```python
from build123d import *

# Parameters (mm, degrees)
BOSS_EXTRUDE1_DEPTH = 65
BOSS_EXTRUDE3_START = -60
SKETCH2_R           = 50
SKETCH2_R_2         = 48
BOSS_EXTRUDE3_DEPTH = 100
CUT_EXTRUDE1_START  = -50
SKETCH2_6_R         = 48
CUT_EXTRUDE1_DEPTH  = 50
BOSS_EXTRUDE6_START = 50
SKETCH2_9_W         = 57.5
SKETCH2_9_H         = 81
SKETCH2_9_W_2       = 53.5
SKETCH2_9_H_2       = 77
BOSS_EXTRUDE6_DEPTH = 100
SKETCH2_10_W        = 53.5
SKETCH2_10_H        = 77
CUT_EXTRUDE2_DEPTH  = 50
SKETCH2_11_W        = 82
SKETCH2_11_H        = 81
SKETCH2_11_W_2      = 78
SKETCH2_11_H_2      = 77
SKETCH2_11_W_3      = 57.5
SKETCH2_11_W_4      = 53.5
SKETCH2_11_R        = 50
SKETCH2_11_R_2      = 48
BOSS_EXTRUDE7_DEPTH = 35
CUT_EXTRUDE4_DEPTH  = 3
SKETCH10_W          = 139.5
SKETCH10_H          = 50
BOSS_EXTRUDE9_DEPTH = 65
SKETCH10_3_W        = 139.5
SKETCH10_3_H        = 50
CUT_EXTRUDE5_DEPTH  = 20
SKETCH7_W           = 139.5
SKETCH7_H           = 50
BOSS_EXTRUDE8_DEPTH = 65
SKETCH8_W           = 135.5
SKETCH8_H           = 65
CUT_EXTRUDE6_DEPTH  = 30


with BuildPart() as part:
    # Sketch1 → Boss-Extrude1 (new body)
    with BuildSketch(Plane(origin=(0, 0, 0), x_dir=(1, 0, 0), z_dir=(0, 1, 0))):
        with BuildLine():
            Line((-70, -50), (120, -50))
            Line((120, -50), (120, 50))
            Line((120, 50), (-71, 50))
            ThreePointArc((-71, 50), (-105.648232278, 35.648232278), (-120, 1))
            Line((-120, 1), (-120, 0))
            ThreePointArc((-120, 0), (-105.355339059, -35.355339059), (-70, -50))
        make_face()
    extrude(amount=BOSS_EXTRUDE1_DEPTH)

    # Sketch2 → Boss-Extrude3 (add)
    with BuildSketch(Plane(origin=(0, 65, 0), x_dir=(1, 0, 0), z_dir=(0, 1, 0)).offset(BOSS_EXTRUDE3_START)):
        with Locations(Location((-70, 0, 0), (0, 0, 270))):
            Circle(SKETCH2_R)
        with Locations(Location((-70, 0, 0), (0, 0, 270))):
            Circle(SKETCH2_R_2, mode=Mode.SUBTRACT)
    extrude(amount=BOSS_EXTRUDE3_DEPTH)

    # Sketch2_6 → Cut-Extrude1 (cut)
    with BuildSketch(Plane(origin=(0, 65, 0), x_dir=(1, 0, 0), z_dir=(0, 1, 0)).offset(CUT_EXTRUDE1_START)):
        with Locations(Location((-70, 0, 0), (0, 0, 270))):
            Circle(SKETCH2_6_R)
    extrude(amount=CUT_EXTRUDE1_DEPTH, mode=Mode.SUBTRACT)

    # Sketch2_9 → Boss-Extrude6 (add)
    with BuildSketch(Plane(origin=(0, 65, 0), x_dir=(1, 0, 0), z_dir=(0, 1, 0)).offset(BOSS_EXTRUDE6_START)):
        with Locations((9.25, 9.5)):
            Rectangle(SKETCH2_9_W, SKETCH2_9_H)
        with Locations((9.25, 9.5)):
            Rectangle(SKETCH2_9_W_2, SKETCH2_9_H_2, mode=Mode.SUBTRACT)
    extrude(amount=-BOSS_EXTRUDE6_DEPTH)

    # Sketch2_10 → Cut-Extrude2 (cut)
    with BuildSketch(Plane(origin=(0, 65, 0), x_dir=(1, 0, 0), z_dir=(0, 1, 0))):
        with Locations((9.25, 9.5)):
            Rectangle(SKETCH2_10_W, SKETCH2_10_H)
    extrude(amount=-CUT_EXTRUDE2_DEPTH, mode=Mode.SUBTRACT)

    # Sketch2_11 → Boss-Extrude7 (add)
    # profile 1 of 3: a face of its own
    with BuildSketch(Plane(origin=(0, 65, 0), x_dir=(1, 0, 0), z_dir=(0, 1, 0))):
        with Locations((79, 9.5)):
            Rectangle(SKETCH2_11_W, SKETCH2_11_H)
        with Locations((79, 9.5)):
            Rectangle(SKETCH2_11_W_2, SKETCH2_11_H_2, mode=Mode.SUBTRACT)
    # profile 2 of 3: a face of its own
    with BuildSketch(Plane(origin=(0, 65, 0), x_dir=(1, 0, 0), z_dir=(0, 1, 0))):
        with Locations((9.25, 9.5)):
            Rectangle(SKETCH2_11_W_3, SKETCH2_11_H)
        with Locations((9.25, 9.5)):
            Rectangle(SKETCH2_11_W_4, SKETCH2_11_H_2, mode=Mode.SUBTRACT)
    # profile 3 of 3: a face of its own
    with BuildSketch(Plane(origin=(0, 65, 0), x_dir=(1, 0, 0), z_dir=(0, 1, 0))):
        with Locations(Location((-70, 0, 0), (0, 0, 270))):
            Circle(SKETCH2_11_R)
        with Locations(Location((-70, 0, 0), (0, 0, 270))):
            Circle(SKETCH2_11_R_2, mode=Mode.SUBTRACT)
    extrude(amount=BOSS_EXTRUDE7_DEPTH)

    # Sketch5 → Cut-Extrude4 (cut)
    with BuildSketch(Plane.XY.offset(31)):
        with BuildLine():
            Line((77.611486798, 100), (77.611486798, 89.725450473))
            ThreePointArc((77.611486798, 89.725450473), (80.540418986, 82.654382661), (87.611486798, 79.725450473))
            Line((87.611486798, 79.725450473), (120, 79.725450473))
            Line((120, 79.725450473), (120, 100))
            Line((120, 100), (77.611486798, 100))
        make_face()
    extrude(amount=-CUT_EXTRUDE4_DEPTH, mode=Mode.SUBTRACT)

    # Sketch10 → Boss-Extrude9 (add)
    with BuildSketch(Plane(origin=(0, 65, 0), x_dir=(1, 0, 0), z_dir=(0, 1, 0))):
        with Locations((50.25, -75)):
            Rectangle(SKETCH10_W, SKETCH10_H)
    extrude(amount=-BOSS_EXTRUDE9_DEPTH)

    # Sketch10_3 → Cut-Extrude5 (cut)
    with BuildSketch(Plane(origin=(0, 65, 0), x_dir=(1, 0, 0), z_dir=(0, 1, 0))):
        with Locations((50.25, -75)):
            Rectangle(SKETCH10_3_W, SKETCH10_3_H)
    extrude(amount=-CUT_EXTRUDE5_DEPTH, mode=Mode.SUBTRACT)

    # Sketch7 → Boss-Extrude8 (add)
    with BuildSketch(Plane(origin=(0, 65, 0), x_dir=(1, 0, 0), z_dir=(0, 1, 0))):
        with Locations((50.25, -75)):
            Rectangle(SKETCH7_W, SKETCH7_H)
    extrude(amount=-BOSS_EXTRUDE8_DEPTH)

    # Sketch8 → Cut-Extrude6 (cut)
    with BuildSketch(Plane(origin=(0, 65, 0), x_dir=(1, 0, 0), z_dir=(0, 1, 0))):
        with Locations((50.25, -65.5)):
            Rectangle(SKETCH8_W, SKETCH8_H)
    extrude(amount=-CUT_EXTRUDE6_DEPTH, mode=Mode.SUBTRACT)


solid = part.part
```
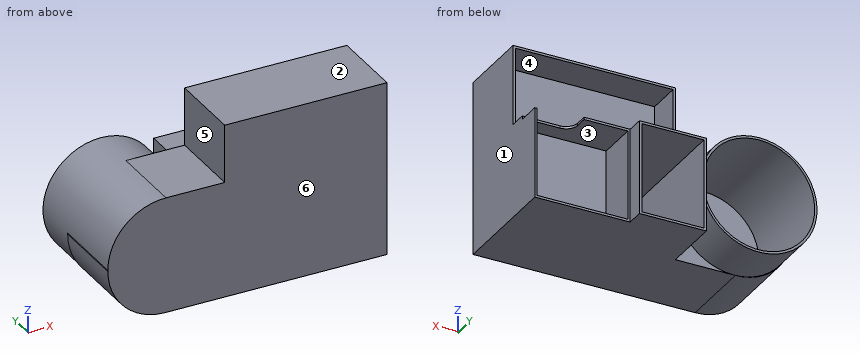
Input: part model. Units: mm. Frame: model coordinates. Face numbers are marked on the shaded views. A direction names the side the tool comes from. Coordinates: 2 decimals unless noted, no trailing zeros. Loops run counter-clockwise (first coordinate to the right, second up) from the corner with the lowest first, then second, coordinate; pieces in that order, holes last. Notation, with made-up numbers: (46, 48.25) - (50, 48.25) arc R15 cw to (50, 67.25) - close; hole circle Ø3 at (59, -5.5). An arc over 180 degrees is marked (long way). Answer in a Markdown table with one row per item.
(1) Material intervals for L1, parallel to X at y = 84.5, z = 0; L2, parallel to X at y = 44, z = 0; L3, parallel to Z at x = 6.5, y = 48, sorted ascending. Write a range as from..to.
Model answer:
| item | result |
|---|---|
| L1 | x = -120..-118, -22..-20, -19.5..-17.5, 36..40, 118..120 |
| L2 | x = -120..-118, -22..-17.5, 36..120 |
| L3 | z = -50..-48, 29..33, 98..100 |
(2) Cut plane C-C on z = -29. Output: boundary loops of the cut face in (x, y).
Model answer:
| item | result |
|---|---|
| outline | (-111.21, 0) - (120, 0) - (120, 100) - (118, 100) - (118, 65) - (40, 65) - (40, 100) - (38, 100) - (38, 115) - (36, 115) - (36, 15) - (-17.5, 15) - (-17.5, 115) - (-19.5, 115) - (-19.5, 65) - (-29.27, 65) - (-29.27, 105) - (-31.75, 105) - (-31.75, 15) - (-108.25, 15) - (-108.25, 105) - (-110.73, 105) - (-110.73, 65) - (-111.21, 65) - close |
(3) Set-up query: the marked faces 4, 5 and 6. Return all of +Z, -Z, +X, -X, +Y, -Y with unobstructed straight access to the full face (end or side cutting, diameter ignored); none if empty.
Model answer:
| item | result |
|---|---|
| face 4 | +Y |
| face 5 | +Z, -X, +Y, -Y |
| face 6 | +Z, -Z, +X, -X, -Y |
(4) Cut plane A-A on y = 50. Output: boundary loops of the cut face in (x, z), plus the area to 3 significant figures.
Model answer:
| item | result |
|---|---|
| outline | (-120, -1) arc R49 ccw to (-71, -50) - (120, -50) - (120, 100) - (-19.5, 100) - (-19.5, 50) - (-70, 50) arc R50 ccw to (-120, 0) - close; hole circle Ø96 at (-70, 0); hole (-17.5, -48) - (36, -48) - (36, 29) - (-17.5, 29) - close; hole (-17.5, 33) - (118, 33) - (118, 98) - (-17.5, 98) - close |
| area | 9,760 mm² |
(5) Mould query, pull axis Z, two halves, no side actions, for the marked faces 1, 2 and 3. Classes: pulls with the +Z half, pulls with the -Z half, needs draft (parallel to the pull), parting line crosses it, or undercut.
Model answer:
| item | result |
|---|---|
| face 1 | needs draft |
| face 2 | pulls with the +Z half |
| face 3 | undercut |
(6) Cut plane B-B on x = 3.5. Output: boundary loops of the cut face in (y, z), plus the area to 3 significant figures.
Model answer:
| item | result |
|---|---|
| outline | (0, -50) - (115, -50) - (115, -48) - (15, -48) - (15, 29) - (115, 29) - (115, 31) - (65, 31) - (65, 33) - (35, 33) - (35, 98) - (65, 98) - (65, 100) - (0, 100) - close |
| area | 4,150 mm² |
(7) Pin query (flat end, axial travel): P1, Ø9, axis at y = 42.5, z = 78.5, coming from the -X side; P2, Ø1, axis at x = -61.5, y = 94, coming from the -Z side; P3, Ø24.5, axis at x = 86.5, z = -4, coming from the +Y side. Return the tip coordinate at first contact, or that it passes through.
Model answer:
| item | result |
|---|---|
| P1 | stops at x = -19.5 |
| P2 | stops at z = -49.36 |
| P3 | stops at y = 65 |
(8) Cut plane D-D on x = -64. Output: boundary loops of the cut face in (y, z).
Model answer:
| item | result |
|---|---|
| outline | (0, -50) - (65, -50) - (65, -49.64) - (105, -49.64) - (105, -47.62) - (15, -47.62) - (15, 47.62) - (105, 47.62) - (105, 49.64) - (65, 49.64) - (65, 50) - (0, 50) - close |
